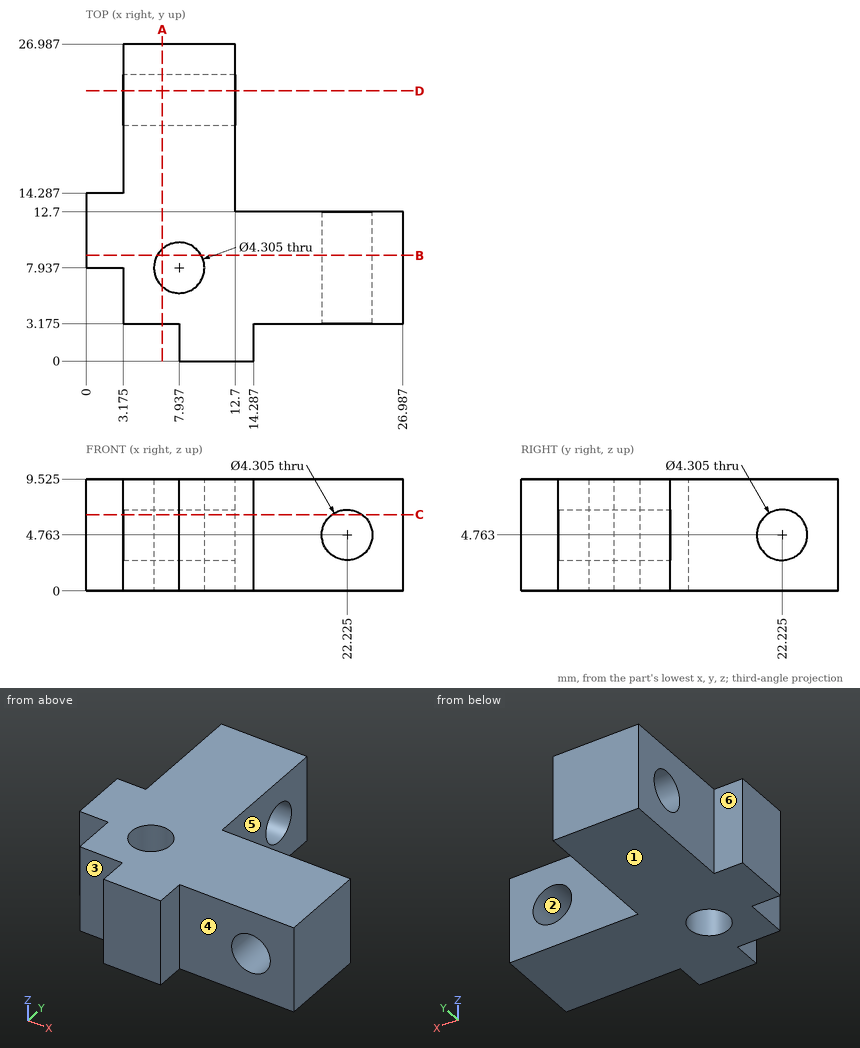
Job drawing, mm, ordinate dimensions from the low corner. One solid piece. A direction names the side the tool comes from. Round coordinates to 2 decimals unless told otherwise and drop trailing zeros. Order: outer loops, then holes, each group sorted by start corner. A loop starts at its lowest first (then second) coordinate and runs counter-clockwise, first axis right, second up. Notation, with made-up numbers: (14, 62.25) - (65, 62.25) arc R15 cw to (65, 67.25) - close; hole circle Ø4 at (29, -10). An arc over 180 degrees is marked (long way). Use CSV: the item, a comma, the result in double quotes. Start each with the question number.
1) Saw through at D-D (y = 23). List the corners of the cut face in (x, z) (1 decimal).
2) Saw through at B-B (y = 9). List the corners of the cut face in (x, z) (1 decimal), and give its area (3 significant figures).
3) Wall check: L1, parallel to X at y = 3.75, z = 1.25 (1 decimal); L2, parallel to Y at x = 19, z = 5.25 (1 decimal); L3, parallel to Y at x = 12.5, z = 6.5 (1 decimal). Give the ranges that are in metal, low to high. Write a range as [from, to].
4) Two-plate mould, pull along Z, no slides. Class the marked faces 1, 2 and 3: pulls with the +Z half, pulls with the -Z half, needs draft (parallel to the pull), parting line crosses it, or undercut.
5) Pin check, flat tips, straight feed: pin 1 Ø1.6 at (x, z) = (1, 5.5) entering from +Y; pin 2 Ø5 at (y, z) = (17.5, 5) entering from +X; pin 3 Ø2.5 at (y, z) = (6, 3.5) entering from -X (1 decimal); pin 4 Ø4 at (x, y) = (7.94, 7.94) entering from -Z. Stop position of each tip, or through.
6) Saw through at A-A (x = 6.5). List the corners of the cut face in (y, z) (1 decimal).
7) Tool access for the marked faces 4, 5 and 6: list every direction of +Z, -Z, +X, -X, +Y, -Y with a clear straight run to the whole face (end or side of a thin tool).
8) Saw through at C-C (z = 6.5). List the corners of the cut face in (x, y) (1 decimal), and give its area (3 significant figures).
Values follow:
1,outline,"(3.2, 0) - (12.7, 0) - (12.7, 2.8) - (3.2, 2.8) - close; (3.2, 6.8) - (12.7, 6.8) - (12.7, 9.5) - (3.2, 9.5) - close"
2,outline,"(0, 0) - (6.1, 0) - (6.1, 9.5) - (0, 9.5) - close; (9.8, 0) - (27, 0) - (27, 9.5) - (9.8, 9.5) - close; hole circle Ø4.3 at (22.2, 4.8)"
2,area,"207 mm2"
3,L1,"x = [3.2, 27]"
3,L2,"y = [3.2, 12.7]"
3,L3,"y = [0, 21], [23.5, 27]"
4,face 1,"pulls with the -Z half"
4,face 2,"undercut"
4,face 3,"needs draft"
5,pin 1,"stops at y = 14.29"
5,pin 2,"stops at x = 12.7"
5,pin 3,"stops at x = 3.2"
5,pin 4,"passes through"
6,outline,"(3.2, 0) - (6.3, 0) - (6.3, 9.5) - (3.2, 9.5) - close; (9.5, 0) - (27, 0) - (27, 9.5) - (9.5, 9.5) - close; hole circle Ø4.3 at (22.2, 4.8)"
7,face 4,"+Z, -Z, +X, -Y"
7,face 5,"+Z, -Z, +X, +Y"
7,face 6,"+Z, -Z, -X, +Y"
8,outline,"(0, 7.9) - (3.2, 7.9) - (3.2, 3.2) - (7.9, 3.2) - (7.9, 0) - (14.3, 0) - (14.3, 3.2) - (21, 3.2) - (21, 12.7) - (12.7, 12.7) - (12.7, 21) - (3.2, 21) - (3.2, 14.3) - (0, 14.3) - close; (3.2, 23.5) - (12.7, 23.5) - (12.7, 27) - (3.2, 27) - close; (23.5, 3.2) - (27, 3.2) - (27, 12.7) - (23.5, 12.7) - close; hole circle Ø4.3 at (7.9, 7.9)"
8,area,"340 mm2"
